Autodesk Inventor part; units mm, degrees
ref_plane "YZ Plane" through (0, 0, 0) normal (1, 0, 0) x (0, 1, 0)
ref_plane "XZ Plane" through (0, 0, 0) normal (0, 1, 0) x (-1, 0, 0)
ref_plane "XY Plane" through (0, 0, 0) normal (0, 0, 1) x (1, 0, 0)
sketch "Sketch1" plane through (0, 0, 0) normal (0, 0, 1) x (1, 0, 0)
  line L0 (-12, 0) -> (12, 0)
  line L1 (12, 0) -> (12, 3)
  line L2 (12, 3) -> (10, 3)
  line L3 (10, 3) -> (10, 4)
  line L4 (10, 4) -> (-10, 4)
  line L5 (-10, 4) -> (-10, 3)
  line L6 (-10, 3) -> (-12, 3)
  line L7 (-12, 3) -> (-12, 0)
  point P0 (0, 0)
  point P1 (0, 0)
  dimension "d0" = 24
  dimension "d1" = 6
  dimension "d2" = 8
  dimension "d3" = 2
revolve "Revolution1" add sketch "Sketch1" angle 360 about axis through (-12, 0, 0) along (1, 0, 0)
sketch "Sketch2" plane through (12, 0, 0) normal (1, 0, 0) x (0, 0, -1)
  point P0 (0, 0)
  point P1 (-0.1005, -0.6753)
  point P2 (-0.0327, -0.0508)
hole "Hole1" at (12, -0.0508, 0.0327) direction (-1, 0, 0) diameter 3.242 end up to surface
chamfer "Chamfer1" distance 0.5 angle 45 2 edges at (12, -0.0508, 1.6537) (-12, -0.0508, 1.6537)
properties part number "BaseSupport" material "Steel, Mild"
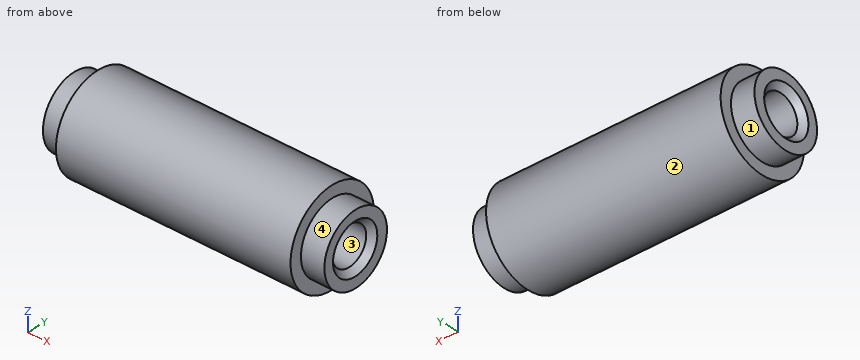
The listing builds one solid part. Answer for the finished solid, in the listing's coordinates (mm). Face numbers are marked on the shaded views. A direction names the side the tool comes from. Round coordinates to 2 decimals unless told otherwise and drop trailing zeros. Write each loop counter-clockwise with the first axis right and the second up, starting at its lowest first coordinate (ties: lowest second). Pieces come first, ordered by that corner, then holes. Notation, with made-up numbers: (76.25, 17.25) -> (128.25, 17.25) arc R21 cw to (128.25, 49.25) -> close; hole circle Ø6 at (87, -27.75). An arc over 180 degrees is marked (long way). Write item = value, one per line.
1) Straight lines are drawn through the part: line 1 along X through (y, z) = (3, -1.5); line 2 along Y through (x, z) = (-7, 1.5); line 3 along Z through (x, y) = (-11, -1). For each, find the intervals that lie inside material, in ascending order. Write a range as [from, to].
Check values:
line_1 = [-10, 10]
line_2 = [-3.71, -0.74], [0.64, 3.71]
line_3 = [-2.83, -1.28], [1.35, 2.83]
2) Section C-C on z = 3.25 is taken. Write down the section's boundary in (x, y), plus the area to 3 significant figures.
Check values:
outline = (-10, -2.33) -> (10, -2.33) -> (10, 2.33) -> (-10, 2.33) -> close
area = 93.3 mm²
3) Section A-A on y = -3.5 is taken. Write down the section's boundary in (x, z).
Check values:
outline = (-10, -1.94) -> (10, -1.94) -> (10, 1.94) -> (-10, 1.94) -> close
4) For a pull along Z with two mould halves and no side action, classify the marked faces 3 and 4 as released by +Z, released by -Z, zero draft, split by the parting line, or undercut.
Check values:
face_3 = undercut
face_4 = split by the parting line
5) Section B-B on x = 4.5 is taken. Write down the section's boundary in (y, z).
Check values:
outline = circle Ø8 at (0, 0); hole circle Ø3.24 at (-0.05, 0.03)
6) Which of the six approach directions +Z, -Z, +X, -X, +Y, -Y give full straight-line access (tool end or side, diameter ignored) to the marked faces 1 and 2?
Check values:
face_1 = -X
face_2 = +X, -X
7) Given pin 1 (3.5 mm diameter, centred on y = -0.05, z = 0.03, fed in from -X); pin 2 (3 mm diameter, centred on x = -1, z = 2.5, fed in from +Y); pin 3 (1.5 mm diameter, centred on x = 5.5, y = 3, fed in from +Z), each flat-ended and moving along its own axis, determine where each tip first touches the part or whether it passes through.
Check values:
pin_1 = -11.63
pin_2 = 3.87
pin_3 = 3.31
